Here's how the part is built. I have some questions about the finished solid (model axes, mm). Face numbers are marked on the shaded views. A direction names the side the tool comes from. Round coordinates to 2 decimals unless told otherwise and drop trailing zeros. Write each loop counter-clockwise with the first axis right and the second up, starting at its lowest first coordinate (ties: lowest second). Pieces come first, ordered by that corner, then holes. Notation, with made-up numbers: (-39.5, 23) -> (15.5, 23) arc R16 ccw to (15.5, 54) -> close; hole circle Ø3 at (78.5, 50.5). An arc over 180 degrees is marked (long way). Answer as CSV lines item,"result".
from build123d import *

# Parameters (mm, degrees)
SKICA1_W                = 2
SKICA1_H                = 30
P_IDAT_VYSUNUT_M1_DEPTH = 40
SKICA2_W                = 4.9
SKICA2_H                = 3
P_IDAT_VYSUNUT_M2_DEPTH = 30
P_IDAT_VYSUNUT_M3_DEPTH = 2


with BuildPart() as part:
    # Skica1 → Přidat vysunutím1 (new body)
    with BuildSketch(Plane.XY):
        with Locations((1, 15)):
            Rectangle(SKICA1_W, SKICA1_H)
    extrude(amount=P_IDAT_VYSUNUT_M1_DEPTH)

    # Skica2 → Přidat vysunutím2 (add)
    with BuildSketch(Plane(origin=(2, 0, 0), x_dir=(0, 0, -1), z_dir=(1, 0, 0))):
        with Locations((-37.55, 28.5)):
            Rectangle(SKICA2_W, SKICA2_H)
        with Locations((-2.45, 28.5)):
            Rectangle(SKICA2_W, SKICA2_H)
        with Locations((-37.55, 23.4)):
            Rectangle(SKICA2_W, SKICA2_H)
        with Locations((-2.45, 23.4)):
            Rectangle(SKICA2_W, SKICA2_H)
    extrude(amount=P_IDAT_VYSUNUT_M2_DEPTH)

    # Skica3 → Přidat vysunutím3 (add)
    with BuildSketch(Plane(origin=(0, 0, 0), x_dir=(-1, 0, 0), z_dir=(0, 0, -1))):
        with BuildLine():
            ThreePointArc((0, 14), (1, 15), (2, 14))
            Line((2, 14), (2, 4))
            ThreePointArc((2, 4), (1, 3), (0, 4))
            Line((0, 4), (0, 1.171572875))
            ThreePointArc((0, 1.171572875), (2.732050808, 1.550510257), (4, 4))
            Line((4, 4), (4, 14))
            ThreePointArc((4, 14), (2.732050808, 16.449489743), (0, 16.828427125))
            Line((0, 16.828427125), (0, 14))
        make_face()
    extrude(amount=-P_IDAT_VYSUNUT_M3_DEPTH)


solid = part.part
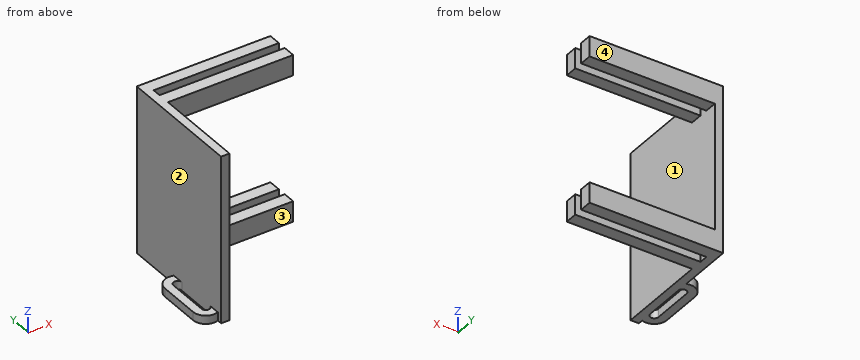
Item 1: I need wall thicknesses on L1, parallel to Y at x = 23.5, z = 37; L2, parallel to Z at x = 26.5, y = 28.5; L3, parallel to X at y = 27.5, z = 34. Which ranges of each line are inside material? Lowest first, please.
Results found:
L1,"y = 21.9 to 24.9, 27 to 30"
L2,"z = 0 to 4.9, 35.1 to 40"
L3,"x = 0 to 2"
Item 2: Suppose I cut it at C-C, the plane x = -1. List the corners of the cut face in (y, z) for me, then the cut area to 3 significant figures.
Results found:
outline,"(1, 0) -> (3, 0) -> (3, 2) -> (1, 2) -> close; (15, 0) -> (17, 0) -> (17, 2) -> (15, 2) -> close"
area,"8.00 mm²"
Item 3: Suppose I cut it at A-A, the plane y = 11. List the corners of the cut face in (x, z) for me.
Results found:
outline,"(-4, 0) -> (-2, 0) -> (-2, 2) -> (-4, 2) -> close; (0, 0) -> (2, 0) -> (2, 40) -> (0, 40) -> close"
Item 4: Suppose I cut it at B-B, the plane x = 24.5. List the corners of the cut face in (y, z) for me.
Results found:
outline,"(21.9, 0) -> (24.9, 0) -> (24.9, 4.9) -> (21.9, 4.9) -> close; (21.9, 35.1) -> (24.9, 35.1) -> (24.9, 40) -> (21.9, 40) -> close; (27, 0) -> (30, 0) -> (30, 4.9) -> (27, 4.9) -> close; (27, 35.1) -> (30, 35.1) -> (30, 40) -> (27, 40) -> close"
Item 5: Suppose I cut it at D-D, the plane y = 24.25. List the corners of the cut face in (x, z) for me, then the cut area to 3 significant figures.
Results found:
outline,"(0, 0) -> (32, 0) -> (32, 4.9) -> (2, 4.9) -> (2, 35.1) -> (32, 35.1) -> (32, 40) -> (0, 40) -> close"
area,"374 mm²"
Item 6: Will these pins go through, and if not, where does the flat tip stop? pin 1 (2 mm diameter, centred on y = 20.5, z = 26.5, fed in from -X); pin 2 (4 mm diameter, centred on x = 12.5, z = 37.5, fed in from -Y); pin 3 (0.6 mm diameter, centred on y = 9, z = 1, fed in from +X).
Results found:
pin 1,"stops at x = 0"
pin 2,"stops at y = 21.9"
pin 3,"stops at x = 2"
Item 7: For the marked faces 3 and 4, which set-ups out of +Z, -Z, +X, -X, +Y, -Y let a thin tool reach every point of the face, with its end or its side?
Results found:
face 3,"+Z, -Z, +X, -Y"
face 4,"+Z, -Z, +X, -X, +Y"
Item 8: If we mould it in two halves opening along Z, with no side actions, what happens to the marked faces 1 and 2? For each: pulls with the +Z half, pulls with the -Z half, needs draft (parallel to the pull), parting line crosses it, or undercut.
Results found:
face 1,"undercut"
face 2,"needs draft"
